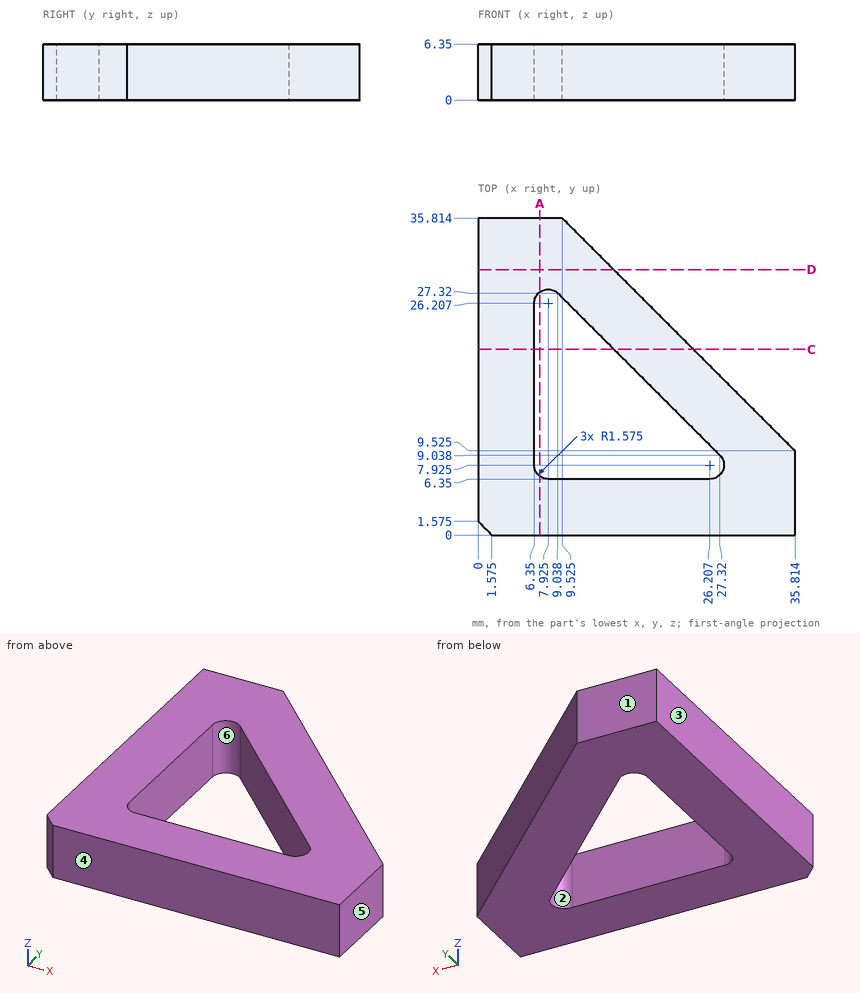
Can you work these out from the drawing? Everything is in mm from the part's minimum corner. A direction names the side the tool comes from. Give positions to 0.01 mm unless a question says otherwise; leave off trailing zeros. Order: outer loops, then holes, each group sorted by start corner. A loop starts at its lowest first (then second) coordinate and runs counter-clockwise, first axis right, second up.
1. For the marked faces 1 and 2, which set-ups out of +Z, -Z, +X, -X, +Y, -Y let a thin tool reach every point of the face, with its end or its side?
2. Will these pins go through, and if not, where does the flat tip stop? P1, Ø1.9, axis at x = 20, z = 2.5, coming from the +Y side; P2, Ø3, axis at y = 16.5, z = 5, coming from the +X side; P3, Ø3, axis at x = 28, z = 0.5, coming from the +Y side.
3. Suppose I cut it at D-D (y = 30). List the corners of the cut face in (x, z) for me.
4. Suppose I cut it at A-A (x = 7). List the corners of the cut face in (y, z) for me.
5. Suppose I cut it at C-C (y = 21). List the corners of the cut face in (x, z) for me.
6. We'd pull the mould along X, two halves only. Please class the marked faces 3, 4, 5 and 6: pulls with the +X half, pulls with the -X half, needs draft (parallel to the pull), parting line crosses it, or undercut.
7. I need wall thicknesses on L1, parallel to Y at x = 8, z = 2; L2, parallel to X at y = 10.5, z = 0.75; L3, parallel to X at y = 26.5, z = 2.5. Which ranges of each line are inside material? Lowest first, please.
Solved:
1. face 1: +Z, -Z, +X, -X, +Y
1. face 2: +Z, -Z
2. P1: stops at y = 26.29
2. P2: stops at x = 30.34
2. P3: stops at y = 18.84
3. outline: (0, 0) - (15.34, 0) - (15.34, 6.35) - (0, 6.35) - close
4. outline: (0, 0) - (6.65, 0) - (6.65, 6.35) - (0, 6.35) - close; (27.48, 0) - (35.81, 0) - (35.81, 6.35) - (27.48, 6.35) - close
5. outline: (0, 0) - (6.35, 0) - (6.35, 6.35) - (0, 6.35) - close; (15.36, 0) - (24.34, 0) - (24.34, 6.35) - (15.36, 6.35) - close
6. face 3: pulls with the -X half
6. face 4: needs draft
6. face 5: pulls with the +X half
6. face 6: undercut
7. L1: y = 0 to 6.35, 27.78 to 35.81
7. L2: x = 0 to 6.35, 25.86 to 34.84
7. L3: x = 0 to 6.38, 9.86 to 18.84
